Autodesk Inventor part; units mm, degrees
ref_plane "YZ Plane" through (0, 0, 0) normal (1, 0, 0) x (0, 1, 0)
ref_plane "XZ Plane" through (0, 0, 0) normal (0, 1, 0) x (-1, 0, 0)
ref_plane "XY Plane" through (0, 0, 0) normal (0, 0, 1) x (1, 0, 0)
sketch "Sketch1" plane through (0, 0, 0) normal (0, 1, 0) x (-1, 0, 0)
  line L0 (28, -25) -> (25, -25)
  line L1 (28, -43) -> (25, -43)
  line L2 (28, -68.5) -> (25, -68.5)
  line L3 (28, -109.5) -> (25, -109.5)
  line L4 (8, -68.5) -> (5, -68.5)
  line L5 (8, -109.5) -> (5, -109.5)
  line L6 (8, -43) -> (5, -43)
  line L7 (8, -25) -> (5, -25)
  line L8 (25, -109.5) -> (25, -68.5)
  line L9 (25, -43) -> (25, -25)
  line L10 (8, -109.5) -> (8, -68.5)
  line L11 (8, -43) -> (8, -25)
  line L12 (8, -160.5) -> (8, -149)
  line L13 (28, -149) -> (25, -149)
  line L14 (8, -149) -> (5, -149)
  line L15 (25, -149) -> (25, -167)
  line L16 (25, -167) -> (28, -167)
  line L17 (5, -167) -> (8.5, -167)
  line L18 (21.5, -169) -> (19.7, -169)
  line L19 (19.7, -169) -> (19.7, -174)
  line L20 (19.7, -174) -> (21.5, -174)
  line L21 (21.5, -174) -> (21.5, -169)
  line L22 (16.5, -110.2512) -> (16.5, -143.2512) construction
  line L23 (28, -25) -> (28, -43)
  line L24 (28, -68.5) -> (28, -109.5)
  line L25 (28, -149) -> (28, -167)
  line L26 (5, -167) -> (5, -149)
  line L27 (5, -109.5) -> (5, -68.5)
  line L28 (5, -43) -> (5, -25)
  line L29 (13, -3) -> (8, -3)
  line L30 (20, -3) -> (20, 0)
  line L31 (20, 0) -> (13, 0)
  line L32 (13, 0) -> (13, -3)
  line L33 (20, -3) -> (25, -3)
  line L34 (4.25, -179) -> (4.25, -182)
  line L35 (11.75, -179) -> (21.25, -179)
  line L36 (21.25, -179) -> (21.25, -182)
  line L37 (21.25, -182) -> (31.0828, -182)
  line L38 (31.25, -179) -> (33, -179)
  line L39 (4.25, -182) -> (2.25, -182)
  line L40 (25, -3) -> (25, 0)
  line L41 (25, 0) -> (30, 0)
  line L42 (8, -3) -> (8, 0)
  line L43 (8, 0) -> (3, 0)
  line L44 (2.25, -185) -> (11.2894, -185)
  arc A0 (31.0828, -182) -> (31.25, -179) centre (4.25, -179) ccw
  arc A1 (5, -141.5838) -> (0, -149) centre (8, -149) ccw
  arc A2 (5, -61.0838) -> (0, -68.5) centre (8, -68.5) ccw
  line L45 (5, -50.4162) -> (5, -61.0838)
  line L46 (5, -116.9162) -> (5, -141.5838)
  line L47 (19.5, -129.25) -> (13.2, -129.25) construction
  arc A3 (0, -109.5) -> (5, -116.9162) centre (8, -109.5) ccw
  line L48 (0, -177.7474) -> (0, -149)
  arc A4 (0, -43) -> (5, -50.4162) centre (8, -43) ccw
  line L49 (0, -109.5) -> (0, -68.5)
  line L50 (0, -43) -> (0, -3)
  arc A5 (33, -54.4564) -> (40.5, -43) centre (28, -43) ccw
  line L51 (40.5, -25) -> (40.5, -43)
  arc A6 (40.5, -25) -> (33, -13.5436) centre (28, -25) ccw
  line L52 (33, -3) -> (33, -13.5436)
  arc A7 (40.5, -149) -> (33, -137.5436) centre (28, -149) ccw
  line L53 (40.5, -167) -> (40.5, -149)
  arc A8 (35.5, -177) -> (40.5, -167) centre (28, -167) ccw
  line L54 (33, -54.4564) -> (33, -137.5436)
  arc A9 (33, -3) -> (30, 0) centre (30, -3) ccw
  arc A10 (3, 0) -> (0, -3) centre (3, -3) ccw
  line L55 (21.5, -144) -> (19.7, -144)
  line L56 (19.7, -144) -> (19.7, -149)
  line L57 (19.7, -149) -> (21.5, -149)
  line L58 (21.5, -149) -> (21.5, -144)
  line L59 (18.5, -160.5) -> (8.5, -160.5)
  line L60 (8.5, -167) -> (8.5, -173.5)
  line L61 (8.5, -173.5) -> (18.5, -173.5)
  line L62 (18.5, -173.5) -> (18.5, -160.5)
  line L63 (13.5, -163.9683) -> (13.5, -168.686) construction
  line L64 (14.8699, -167) -> (11.7199, -167) construction
  arc A11 (11.2894, -185) -> (11.75, -182) centre (1.75, -182) ccw
  line L65 (11.75, -182) -> (11.75, -179)
  line L66 (14.25, -179) -> (14.25, -182) construction
  line L67 (14.25, -182) -> (4.25, -182) construction
  line L68 (31.25, -179) -> (31.25, -182) construction
  line L69 (31.25, -182) -> (31.0828, -182) construction
  line L70 (33, -179) -> (35.5, -179)
  line L71 (35.5, -179) -> (35.5, -177)
  line L72 (33, -179) -> (33, -174.1753) construction
  line L73 (28, -179) -> (28, -186) construction
  line L74 (28, -186) -> (25, -186) construction
  line L75 (25, -186) -> (25, -179) construction
  line L76 (31.25, -179) -> (21.25, -179) construction
  line L77 (4.25, -179) -> (0, -177.7474)
  line L78 (1.75, -182.5) -> (1.75, -184.5)
  arc A12 (2.25, -182) -> (1.75, -182.5) centre (2.25, -182.5) ccw
  arc A13 (1.75, -184.5) -> (2.25, -185) centre (2.25, -184.5) ccw
  line L79 (8.5, -160.5) -> (8, -160.5)
  line L80 (26.5, -73.5989) -> (26.5, -105.0523) construction
  line L81 (6.5, -72.0232) -> (6.5, -105.7187) construction
  point P0 (0, 0)
  point P1 (1.75, -185)
  dimension "d7" = 18
  dimension "d8" = 25.5
  dimension "d9" = 41
  dimension "d39" = 18
  dimension "d45" = 5
  dimension "d56" = 3
  dimension "d61" = 39.5
  dimension "d64" = 12
  dimension "d65" = 7
  dimension "d74" = 176
  dimension "d75" = 17
  dimension "d85" = 10
  dimension "d90" = 5
  dimension "d92" = 25
  dimension "d104" = 6
  dimension "d105" = 5
  dimension "d106" = 1.8
  dimension "d107" = 3.5
  dimension "d108" = 20
  dimension "d112" = 8
  dimension "d113" = 12
  dimension "d114" = 7
  dimension "d115" = 10
  dimension "d116" = 3
  dimension "d121" = 2.5
  dimension "d122" = 25
  dimension "d123" = 7
  dimension "d124" = 10
  dimension "d125" = 2.5
  dimension "d126" = 2.5
  dimension "d127" = 0.5
  dimension "d129" = 13
  dimension "d130" = 10
  dimension "d134" = 17
extrude "Extrusion3" add sketch "Sketch1" along normal blind 3
properties part number "Left_wall"
The listing builds one solid part. Answer for the finished solid, in the listing's coordinates (mm). A direction names the side the tool comes from. Round coordinates to 2 decimals unless told otherwise and drop trailing zeros. Write each loop counter-clockwise with the first axis right and the second up, starting at its lowest first coordinate (ties: lowest second). Pieces come first, ordered by that corner, then holes. Notation, with made-up numbers: M -24,-25.5 L 31,-25.5 A25 cw 31,11.5 Z; hole C 37.5,47.25 d9. An arc over 180 degrees is marked long. Write each question's results on one line, items separated by ' | '. Start each with the question number.
Item 1: For a pull along Z with two mould halves and no side action, classify faces 5 (the face through (-40.5, 1, -34)), 6 (the face through (-31.21, 1.48, -180.48)), 7 (the face through (-7, 1, -68.5)) as pulls with the +Z half, pulls with the -Z half, needs draft (parallel to the pull), parting line crosses it, or undercut.
Item 2: Flat-ended cylindrical pins translate along their axes: pin 1 Ø0.9 at (y, z) = (2, -181) entering from +X; pin 2 Ø1.5 at (x, y) = (-26, 1) entering from -Z; pin 3 Ø1.5 at (y, z) = (2, -146) entering from +X. Find the tip coordinate at first contact, or state that the pin passes through.
Item 3: For faces 1 (the face through (-16, 1, -179)), 2 (the face through (-19.7, 1, -171)), 3 (the face through (-1.404, 1.479, -47.527)), 4 (the face through (-11, 1, -3)), determine the directions among +Z, -Z, +X, -X, +Y, -Y from which every point of the face is accessible in a straight line to the end or side of a thin tool.
Item 4: A cutting plane is placed at B-B on z = -146. Write down the section's boundary in (x, y).
Item 5: A cutting plane is placed at C-C on y = 0.8. State how many separate pieces and enclosed holes the cut face has, and give its area (3 significant figures).
Item 6: Straight lines are drawn through the part: L1, parallel to X at y = 0.3, z = -153.5; L2, parallel to X at y = 1.8, z = -81.5; L3, parallel to Z at x = -27.5, y = 2.7. For each, find the intervals that lie inside material, in ascending order. Write a range as [from, to].
Item 7: A cutting plane is placed at A-A on x = -15.5. Write down the section's boundary in (y, z).
Check sheet entries:
1) face 5: needs draft | face 6: pulls with the -Z half | face 7: undercut
2) pin 1: x = -4.25 | pin 2: z = -182 | pin 3: x = -0.32
3) face 1: -Z, +Y, -Y | face 2: +Y, -Y | face 3: +X, +Y, -Y | face 4: +Z, +Y, -Y
4) outline: M -40.13,0 L -21.5,0 L -21.5,3 L -40.13,3 Z; M -19.7,0 L -0.58,0 L -0.58,3 L -19.7,3 Z
5) separate pieces: 1 | enclosed holes: 8 | area: 5,640 mm²
6) L1: [-40.5, -28], [-25, -8], [-5, 0] | L2: [-33, -28], [-25, -8], [-5, 0] | L3: [-182, -167], [-149, -109.5], [-68.5, -43], [-25, 0]
7) outline: M 0,-179 L 3,-179 L 3,-173.5 L 0,-173.5 Z; M 0,-160.5 L 3,-160.5 L 3,0 L 0,0 Z
